```python
from build123d import *

# Parameters (mm, degrees)
F0_R     = 5
F1_DEPTH = 3


# Not quite as in the source:
# - a feature names something its author has since deleted; it is built from what else it names


with BuildPart() as f1:
    # F0 (on Top) → F1 (new body)
    with BuildSketch(Plane.XY):
        with BuildLine():
            Line((65, 30), (65, 40))
            Line((65, 40), (55, 40))
            Line((55, 40), (55, 34.3301270189))
            ThreePointArc((55, 34.3301270189), (56.8301270189, 32.5), (57.5, 30))
            Line((57.5, 30), (65, 30))
        make_face()
        with BuildLine():
            Line((55, 34.3301270189), (55, 40))
            Line((55, 40), (-55.1096590387, 40))
            Line((-55.1096590387, 40), (-55.1096590387, 34.2649360724))
            ThreePointArc((-55.1096590387, 34.2649360724), (-50.0554443342, 34.3616679833), (-47.5, 30))
            Line((-47.5, 30), (-42.5, 30))
            ThreePointArc((-42.5, 30), (-37.5, 35), (-32.5, 30))
            Line((-32.5, 30), (-27.5, 30))
            ThreePointArc((-27.5, 30), (-22.5, 35), (-17.5, 30))
            Line((-17.5, 30), (-12.5, 30))
            ThreePointArc((-12.5, 30), (-7.5, 35), (-2.5, 30))
            Line((-2.5, 30), (2.5, 30))
            ThreePointArc((2.5, 30), (7.5, 35), (12.5, 30))
            Line((12.5, 30), (17.5, 30))
            ThreePointArc((17.5, 30), (22.5, 35), (27.5, 30))
            Line((27.5, 30), (32.5, 30))
            ThreePointArc((32.5, 30), (37.5, 35), (42.5, 30))
            Line((42.5, 30), (47.5, 30))
            ThreePointArc((47.5, 30), (50, 34.3301270189), (55, 34.3301270189))
        make_face()
        with BuildLine():
            Line((65, -30), (65, 30))
            Line((65, 30), (57.5, 30))
            ThreePointArc((57.5, 30), (56.8301270189, 27.5), (55, 25.6698729811))
            Line((55, 25.6698729811), (55, 19.3301270189))
            ThreePointArc((55, 19.3301270189), (56.8301270189, 17.5), (57.5, 15))
            ThreePointArc((57.5, 15), (56.8301270189, 12.5), (55, 10.6698729811))
            Line((55, 10.6698729811), (55, 4.3301270189))
            ThreePointArc((55, 4.3301270189), (56.8301270189, 2.5), (57.5, 0))
            ThreePointArc((57.5, 0), (56.8301270189, -2.5), (55, -4.3301270189))
            Line((55, -4.3301270189), (55, -10.6698729811))
            ThreePointArc((55, -10.6698729811), (56.8301270189, -12.5), (57.5, -15))
            ThreePointArc((57.5, -15), (56.8301270189, -17.5), (55, -19.3301270189))
            Line((55, -19.3301270189), (55, -25.6698729811))
            ThreePointArc((55, -25.6698729811), (56.8301270189, -27.5), (57.5, -30))
            Line((57.5, -30), (65, -30))
        make_face()
        with BuildLine():
            Line((-55.1096590387, 34.2649360724), (-55.1096590387, 40))
            Line((-55.1096590387, 40), (-65, 40))
            Line((-65, 40), (-65, 30))
            Line((-65, 30), (-57.5, 30))
            ThreePointArc((-57.5, 30), (-56.8616679833, 32.4445556658), (-55.1096590387, 34.2649360724))
        make_face()
        with BuildLine():
            Line((65, -40), (65, -30))
            Line((65, -30), (57.5, -30))
            ThreePointArc((57.5, -30), (56.8301270189, -32.5), (55, -34.3301270189))
            Line((55, -34.3301270189), (55, -40))
            Line((55, -40), (65, -40))
        make_face()
        with BuildLine():
            ThreePointArc((55, 25.6698729811), (50, 25.6698729811), (47.5, 30))
            Line((47.5, 30), (42.5, 30))
            ThreePointArc((42.5, 30), (37.5, 25), (32.5, 30))
            Line((32.5, 30), (27.5, 30))
            ThreePointArc((27.5, 30), (22.5, 25), (17.5, 30))
            Line((17.5, 30), (12.5, 30))
            ThreePointArc((12.5, 30), (7.5, 25), (2.5, 30))
            Line((2.5, 30), (-2.5, 30))
            ThreePointArc((-2.5, 30), (-7.5, 25), (-12.5, 30))
            Line((-12.5, 30), (-17.5, 30))
            ThreePointArc((-17.5, 30), (-22.5, 25), (-27.5, 30))
            Line((-27.5, 30), (-32.5, 30))
            ThreePointArc((-32.5, 30), (-37.5, 25), (-42.5, 30))
            Line((-42.5, 30), (-47.5, 30))
            ThreePointArc((-47.5, 30), (-50.0554443342, 25.6383320167), (-55.1096590387, 25.7350639276))
            Line((-55.1096590387, 25.7350639276), (-55.1096590387, 19.2649360724))
            ThreePointArc((-55.1096590387, 19.2649360724), (-50.0554443342, 19.3616679833), (-47.5, 15))
            ThreePointArc((-47.5, 15), (-50.0554443342, 10.6383320167), (-55.1096590387, 10.7350639276))
            Line((-55.1096590387, 10.7350639276), (-55.1096590387, 4.2649360724))
            ThreePointArc((-55.1096590387, 4.2649360724), (-50.0554443342, 4.3616679833), (-47.5, 0))
            ThreePointArc((-47.5, 0), (-50.0554443342, -4.3616679833), (-55.1096590387, -4.2649360724))
            Line((-55.1096590387, -4.2649360724), (-55.1096590387, -10.7350639276))
            ThreePointArc((-55.1096590387, -10.7350639276), (-50.0554443342, -10.6383320167), (-47.5, -15))
            ThreePointArc((-47.5, -15), (-50.0554443342, -19.3616679833), (-55.1096590387, -19.2649360724))
            Line((-55.1096590387, -19.2649360724), (-55.1096590387, -25.7350639276))
            ThreePointArc((-55.1096590387, -25.7350639276), (-50.0554443342, -25.6383320167), (-47.5, -30))
            Line((-47.5, -30), (-42.5, -30))
            ThreePointArc((-42.5, -30), (-37.5, -25), (-32.5, -30))
            Line((-32.5, -30), (-27.5, -30))
            ThreePointArc((-27.5, -30), (-22.5, -25), (-17.5, -30))
            Line((-17.5, -30), (-12.5, -30))
            ThreePointArc((-12.5, -30), (-7.5, -25), (-2.5, -30))
            Line((-2.5, -30), (2.5, -30))
            ThreePointArc((2.5, -30), (7.5, -25), (12.5, -30))
            Line((12.5, -30), (17.5, -30))
            ThreePointArc((17.5, -30), (22.5, -25), (27.5, -30))
            Line((27.5, -30), (32.5, -30))
            ThreePointArc((32.5, -30), (37.5, -25), (42.5, -30))
            Line((42.5, -30), (47.5, -30))
            ThreePointArc((47.5, -30), (50, -25.6698729811), (55, -25.6698729811))
            Line((55, -25.6698729811), (55, -19.3301270189))
            ThreePointArc((55, -19.3301270189), (47.5, -15), (55, -10.6698729811))
            Line((55, -10.6698729811), (55, -4.3301270189))
            ThreePointArc((55, -4.3301270189), (47.5, 0), (55, 4.3301270189))
            Line((55, 4.3301270189), (55, 10.6698729811))
            ThreePointArc((55, 10.6698729811), (47.5, 15), (55, 19.3301270189))
            Line((55, 19.3301270189), (55, 25.6698729811))
        make_face()
        with Locations((-37.5, -15)):
            Circle(F0_R, mode=Mode.SUBTRACT)
        with Locations((-22.5, -15)):
            Circle(F0_R, mode=Mode.SUBTRACT)
        with Locations((-7.5, -15)):
            Circle(F0_R, mode=Mode.SUBTRACT)
        with Locations((-37.5, 0)):
            Circle(F0_R, mode=Mode.SUBTRACT)
        with Locations((-22.5, 0)):
            Circle(F0_R, mode=Mode.SUBTRACT)
        with Locations((-7.5, 0)):
            Circle(F0_R, mode=Mode.SUBTRACT)
        with Locations((7.5, -15)):
            Circle(F0_R, mode=Mode.SUBTRACT)
        with Locations((22.5, -15)):
            Circle(F0_R, mode=Mode.SUBTRACT)
        with Locations((7.5, 0)):
            Circle(F0_R, mode=Mode.SUBTRACT)
        with Locations((22.5, 0)):
            Circle(F0_R, mode=Mode.SUBTRACT)
        with Locations((37.5, -15)):
            Circle(F0_R, mode=Mode.SUBTRACT)
        with Locations((37.5, 0)):
            Circle(F0_R, mode=Mode.SUBTRACT)
        with Locations((-37.5, 15)):
            Circle(F0_R, mode=Mode.SUBTRACT)
        with Locations((-22.5, 15)):
            Circle(F0_R, mode=Mode.SUBTRACT)
        with Locations((-7.5, 15)):
            Circle(F0_R, mode=Mode.SUBTRACT)
        with Locations((7.5, 15)):
            Circle(F0_R, mode=Mode.SUBTRACT)
        with Locations((22.5, 15)):
            Circle(F0_R, mode=Mode.SUBTRACT)
        with Locations((37.5, 15)):
            Circle(F0_R, mode=Mode.SUBTRACT)
        with BuildLine():
            Line((-57.5, 30), (-65, 30))
            Line((-65, 30), (-65, -30))
            Line((-65, -30), (-57.5, -30))
            ThreePointArc((-57.5, -30), (-56.8616679833, -27.5554443342), (-55.1096590387, -25.7350639276))
            Line((-55.1096590387, -25.7350639276), (-55.1096590387, -19.2649360724))
            ThreePointArc((-55.1096590387, -19.2649360724), (-57.5, -15), (-55.1096590387, -10.7350639276))
            Line((-55.1096590387, -10.7350639276), (-55.1096590387, -4.2649360724))
            ThreePointArc((-55.1096590387, -4.2649360724), (-57.5, 0), (-55.1096590387, 4.2649360724))
            Line((-55.1096590387, 4.2649360724), (-55.1096590387, 10.7350639276))
            ThreePointArc((-55.1096590387, 10.7350639276), (-57.5, 15), (-55.1096590387, 19.2649360724))
            Line((-55.1096590387, 19.2649360724), (-55.1096590387, 25.7350639276))
            ThreePointArc((-55.1096590387, 25.7350639276), (-56.8616679833, 27.5554443342), (-57.5, 30))
        make_face()
        with BuildLine():
            Line((-55.1096590387, -40), (55, -40))
            Line((55, -40), (55, -34.3301270189))
            ThreePointArc((55, -34.3301270189), (50, -34.3301270189), (47.5, -30))
            Line((47.5, -30), (42.5, -30))
            ThreePointArc((42.5, -30), (37.5, -35), (32.5, -30))
            Line((32.5, -30), (27.5, -30))
            ThreePointArc((27.5, -30), (22.5, -35), (17.5, -30))
            Line((17.5, -30), (12.5, -30))
            ThreePointArc((12.5, -30), (7.5, -35), (2.5, -30))
            Line((2.5, -30), (-2.5, -30))
            ThreePointArc((-2.5, -30), (-7.5, -35), (-12.5, -30))
            Line((-12.5, -30), (-17.5, -30))
            ThreePointArc((-17.5, -30), (-22.5, -35), (-27.5, -30))
            Line((-27.5, -30), (-32.5, -30))
            ThreePointArc((-32.5, -30), (-37.5, -35), (-42.5, -30))
            Line((-42.5, -30), (-47.5, -30))
            ThreePointArc((-47.5, -30), (-50.0554443342, -34.3616679833), (-55.1096590387, -34.2649360724))
            Line((-55.1096590387, -34.2649360724), (-55.1096590387, -40))
        make_face()
        with BuildLine():
            Line((-57.5, -30), (-65, -30))
            Line((-65, -30), (-65, -40))
            Line((-65, -40), (-55.1096590387, -40))
            Line((-55.1096590387, -40), (-55.1096590387, -34.2649360724))
            ThreePointArc((-55.1096590387, -34.2649360724), (-56.8616679833, -32.4445556658), (-57.5, -30))
        make_face()
    extrude(amount=F1_DEPTH)


solid = f1.part
```
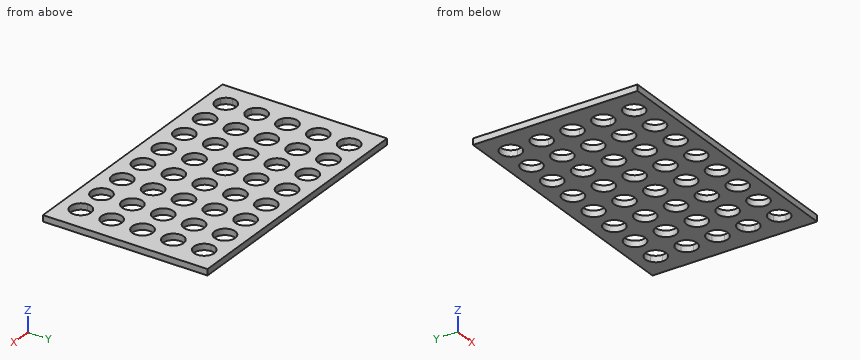
Geometry check sheet. Reference: the model listing, model coordinates, mm. Coordinates: 2 decimals unless noted, no trailing zeros. Order: outer loops, then holes, each group sorted by start corner. A loop starts at its lowest first (then second) coordinate and runs counter-clockwise, first axis right, second up.
Item 1: Section check A-A (x = 22.5). Enter the section's corners in (y, z), plus the area to 3 significant figures.
Item 2: Section check C-C (x = 36.5). Enter the section's corners in (y, z), plus the area to 3 significant figures.
Item 3: Section check B-B (z = 0.75). Count the separate pieces of the cut face and the enclosed holes in it, plus the area to 3 significant figures.
Item 4: Scan lines: line 1 along Y through (x, z) = (52, 0.4); line 2 along Y through (x, z) = (-3, 2.5). Record each from-to range of solid material in increasing order.
Check sheet entries:
1. outline: (-40, 0) - (-35, 0) - (-35, 3) - (-40, 3) - close; (-25, 0) - (-20, 0) - (-20, 3) - (-25, 3) - close; (-10, 0) - (-5, 0) - (-5, 3) - (-10, 3) - close; (5, 0) - (10, 0) - (10, 3) - (5, 3) - close; (20, 0) - (25, 0) - (25, 3) - (20, 3) - close; (35, 0) - (40, 0) - (40, 3) - (35, 3) - close
1. area: 90.0 mm2
2. outline: (-40, 0) - (-34.9, 0) - (-34.9, 3) - (-40, 3) - close; (-25.1, 0) - (-19.9, 0) - (-19.9, 3) - (-25.1, 3) - close; (-10.1, 0) - (-4.9, 0) - (-4.9, 3) - (-10.1, 3) - close; (4.9, 0) - (10.1, 0) - (10.1, 3) - (4.9, 3) - close; (19.9, 0) - (25.1, 0) - (25.1, 3) - (19.9, 3) - close; (34.9, 0) - (40, 0) - (40, 3) - (34.9, 3) - close
2. area: 93.0 mm2
3. separate pieces: 1
3. enclosed holes: 40
3. area: 7,260 mm2
4. line 1: y = -40 to -34.97, -25.03 to -19.97, -10.03 to -4.97, 4.97 to 10.03, 19.97 to 25.03, 34.97 to 40
4. line 2: y = -40 to -32.18, -27.82 to -17.18, -12.82 to -2.18, 2.18 to 12.82, 17.18 to 27.82, 32.18 to 40
